Design review of the part shown in the three views and the two pictorial views. Dimensions are in mm from the part's minimum x, y and z. Coordinates: 2 decimals unless noted, no trailing zeros. Loops run counter-clockwise (first coordinate to the right, second up) from the corner with the lowest first, then second, coordinate; pieces in that order, holes last.
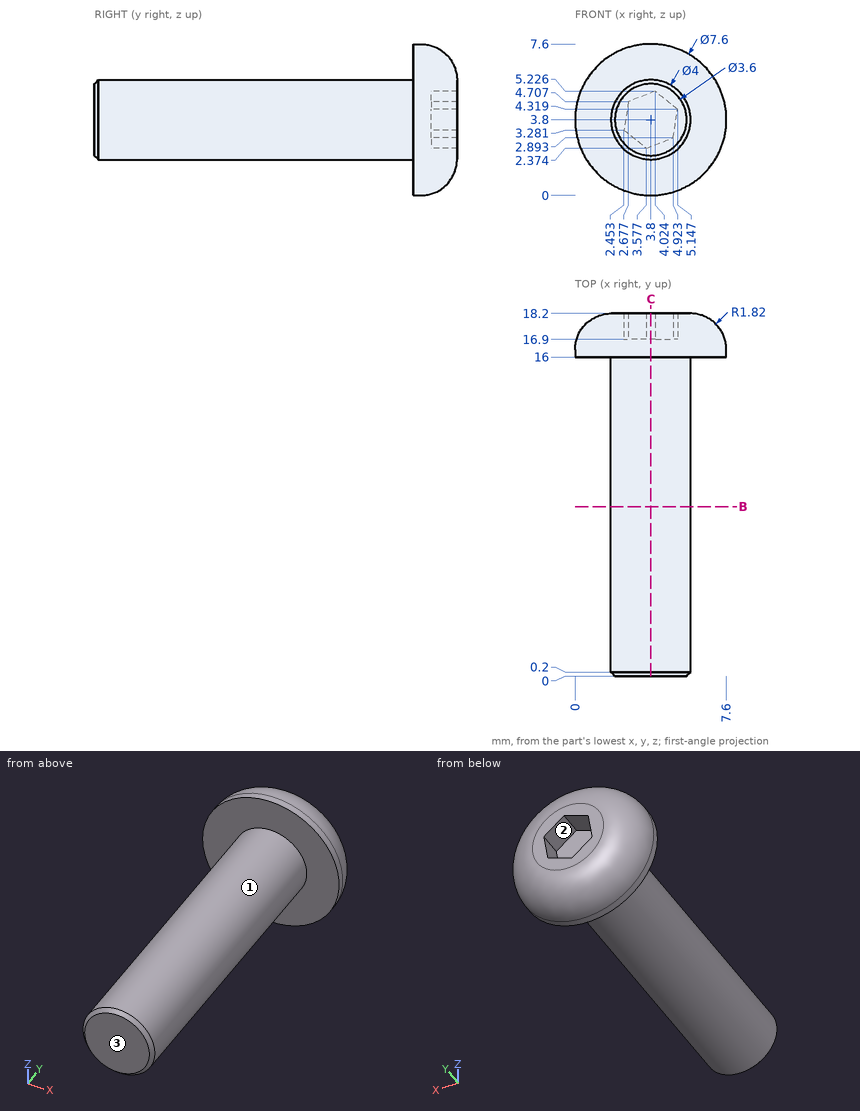
Q1. For pin 1 Ø1 at (y, z) = (3.5, 3.5) entering from -X; pin 2 Ø2 at (x, z) = (1.5, 5.5) entering from -Y; pin 3 Ø1.5 at (x, z) = (4.5, 4.5) entering from -Y; pin 4 Ø4 at (x, y) = (6.5, 8.5) entering from -Z, all flat-tipped, find the tip position at first contact; note any pin that passes through.
Q2. Wall thickness on probe 1 along X at (y, z) = (9, 3.5); probe 2 along Y at (x, z) = (3.5, 3.75): over which ranges is each line inside the solid? List them lowest first.
Q3. Consider section C-C (x = 3.8). State the section outline as (y, z) points.
Q4. The part is to be moulded in two halves that separate along Z. For the marked faces 1, 2 and 3, say which applies: +Z half, -Z half, draft (parallel to the pull), parting line (faces both ways), or undercut.
Q5. Consider section B-B (y = 8.5). State the section outline as (x, z) points, then the cut area to 3 significant figures.
Model answer:
1. pin 1: stops at x = 1.8
1. pin 2: stops at y = 0.06
1. pin 3: stops at y = 0
1. pin 4: stops at z = 1.93
2. probe 1: x = 1.82 to 5.78
2. probe 2: y = 0 to 16.9
3. outline: (0, 2) - (0.2, 1.8) - (16, 1.8) - (16, 0) - (16.38, 0) arc R1.82 ccw to (18.2, 1.82) - (18.2, 2.46) - (16.9, 2.46) - (16.9, 5.14) - (18.2, 5.14) - (18.2, 5.78) arc R1.82 ccw to (16.38, 7.6) - (16, 7.6) - (16, 5.8) - (0.2, 5.8) - (0, 5.6) - close
4. face 1: parting line
4. face 2: undercut
4. face 3: draft
5. outline: circle Ø4 at (3.8, 3.8)
5. area: 12.6 mm2
